from build123d import *

# Parameters (mm, degrees)
SKETCH1_R           = 5
BOSS_EXTRUDE1_DEPTH = 5.5
SKETCH2_R           = 1.75
CUT_EXTRUDE1_DEPTH  = 4
DOME1_FACE_RADIUS   = 5
DOME1_HEIGHT        = 1
FILLET1_R           = 0.5


with BuildPart() as part:
    # Sketch1 → Boss-Extrude1 (new body)
    with BuildSketch(Plane(origin=(0, 0, 0), x_dir=(1, 0, 0), z_dir=(0, 1, 0))):
        with Locations(Location((0, 0, 0), (0, 0, 270))):
            Circle(SKETCH1_R)
    extrude(amount=BOSS_EXTRUDE1_DEPTH)

    # Sketch2 → Cut-Extrude1 (cut)
    with BuildSketch(Plane.XZ):
        with Locations(Location((0, 0, 0), (0, 0, 270))):
            Circle(SKETCH2_R)
    extrude(amount=-CUT_EXTRUDE1_DEPTH, mode=Mode.SUBTRACT)

    # Dome1: a dome of height H over a round flat face of radius A is a cap of a sphere of radius (A * A + H * H) / (2 * H)
    dome1_r = (DOME1_FACE_RADIUS * DOME1_FACE_RADIUS + DOME1_HEIGHT * DOME1_HEIGHT) / (2 * DOME1_HEIGHT)
    dome1_base = Plane((0, 5.5, 0), z_dir=(0, -1, 0))
    with Locations(dome1_base.offset(DOME1_HEIGHT - dome1_r)):
        dome1_ball = Sphere(dome1_r, mode=Mode.PRIVATE)
    add(split(dome1_ball, bisect_by=dome1_base, keep=Keep.TOP, mode=Mode.PRIVATE), mode=Mode.SUBTRACT)

    # Fillet1
    fillet1_edges = [part.edges().sort_by_distance(p)[0] for p in [
        (-5, 5.5, 0),
    ]]
    fillet(fillet1_edges, radius=FILLET1_R)


solid = part.part
Input: part model. Units: mm. Frame: model coordinates. Give positions to 0.01 mm unless a question says otherwise; leave off trailing zeros. Order: outer loops, then holes, each group sorted by start corner. A loop starts at its lowest first (then second) coordinate and runs counter-clockwise, first axis right, second up. Notation, with made-up numbers: M 52,72 L 68,72 A22 ccw 68,98 Z; hole C 80.5,18 d4. An arc over 180 degrees is marked long. Answer as a JSON object with one key per item and string values.
1. Ray query, line 1 (X direction, y = 2.6, z = 0); line 2 (Z direction, x = 1.5, y = 0.55); line 3 (X direction, y = 2.6, z = -1.25). Return the intervals inside material, ascending. Write a range as [from, to].
Result sheet:
{"line 1": "[-5, -1.75], [1.75, 5]", "line 2": "[-4.77, -0.9], [0.9, 4.77]", "line 3": "[-4.84, -1.22], [1.22, 4.84]"}
2. Cut plane B-B, the plane y = 4.2. Output: boundary loops of the cut face in (x, z).
Result sheet:
{"outline": "C 0,0 d10"}
3. First-contact query: P1, Ø1, axis at x = 0, z = 2.5, coming from the +Y side; P2, Ø4.5, axis at x = 0, z = 0, coming from the +Y side. Flat tips, straight axial feed; report the tip coordinate or a pass-through.
Result sheet:
{"P1": "y = 4.85", "P2": "y = 4.7"}
4. Cut plane A-A, the plane y = 3.55. Output: boundary loops of the cut face in (x, z), and give its area (3 significant figures).
Result sheet:
{"outline": "C 0,0 d10; hole C 0,0 d3.5", "area": "68.9 mm²"}
5. Pull-direction query (X, two-part tool) for faces 1 (the cylindrical face through (-4.88, 2.35, -1.08)), 2 (the cylindrical face through (-1.71, 1.97, 0.38)), 3 (the flat face through (0, 4, 0)), 4 (the flat face through (0, 0, 2)); classes: +X half, -X half, draft (parallel to the pull), parting line (faces both ways), or undercut.
Result sheet:
{"face 1": "parting line", "face 2": "undercut", "face 3": "undercut", "face 4": "draft"}
